Job drawing, mm, ordinate dimensions from the low corner. One solid piece. A direction names the side the tool comes from. Give positions to 0.01 mm unless a question says otherwise; leave off trailing zeros. Loops run counter-clockwise (first coordinate to the right, second up) from the corner with the lowest first, then second, coordinate; pieces in that order, holes last. Notation, with made-up numbers: (-24, 25) -> (-2, 25) arc R26 cw to (-2, 46) -> close; hole circle Ø2 at (41, 42). An arc over 180 degrees is marked (long way). Use one line per item in the form item = value.
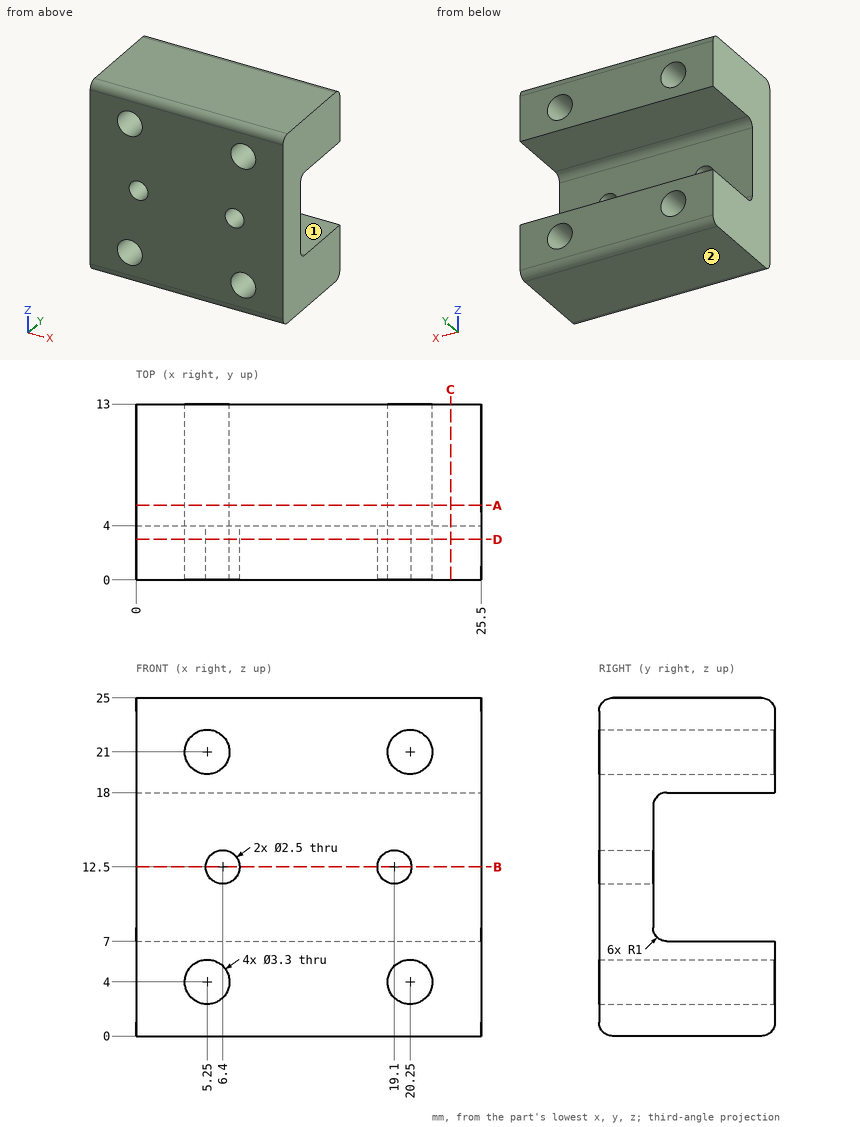
1. Cut at B-B, the plane z = 12.5. Write the cut outline in (x, y), then the cut area to 3 significant figures.
Result sheet:
outline = (0, 0) -> (5.15, 0) -> (5.15, 4) -> (0, 4) -> close; (7.65, 0) -> (17.85, 0) -> (17.85, 4) -> (7.65, 4) -> close; (20.35, 0) -> (25.5, 0) -> (25.5, 4) -> (20.35, 4) -> close
area = 82.0 mm^2
2. Drill centre lines: line 1 (X direction, y = 7, z = 21); line 2 (X direction, y = 12, z = 19.75); line 3 (Z direction, x = 13.5, y = 5.75). Where is each one in solid material? Low to high.
Result sheet:
line_1 = 0 to 3.6, 6.9 to 18.6, 21.9 to 25.5
line_2 = 0 to 4.17, 6.33 to 19.17, 21.33 to 25.5
line_3 = 0 to 7, 18 to 25
3. Cut at A-A, the plane y = 5.5. Write the cut outline in (x, z).
Result sheet:
outline = (0, 0) -> (25.5, 0) -> (25.5, 7) -> (0, 7) -> close; (0, 18) -> (25.5, 18) -> (25.5, 25) -> (0, 25) -> close; hole circle Ø3.3 at (5.25, 4); hole circle Ø3.3 at (5.25, 21); hole circle Ø3.3 at (20.25, 4); hole circle Ø3.3 at (20.25, 21)
4. Tool access for the marked faces 1 and 2: list every direction of +Z, -Z, +X, -X, +Y, -Y with a clear straight run to the whole face (end or side of a thin tool).
Result sheet:
face_1 = +X, -X, +Y
face_2 = -Z, +X, -X, +Y, -Y
5. Cut at C-C, the plane x = 23.25. Write the cut outline in (y, z).
Result sheet:
outline = (0, 1) arc R1 ccw to (1, 0) -> (12, 0) arc R1 ccw to (13, 1) -> (13, 7) -> (5, 7) arc R1 cw to (4, 8) -> (4, 17) arc R1 cw to (5, 18) -> (13, 18) -> (13, 24) arc R1 ccw to (12, 25) -> (1, 25) arc R1 ccw to (0, 24) -> close
6. Drop flat-ended pins along their axis: P1, Ø2.5, axis at x = 5.25, z = 4, coming from the -Y side; P2, Ø1.5, axis at x = 9.5, z = 16.5, coming from the +Y side; P3, Ø7, axis at x = 8, z = 14, coming from the +Y side. Give the stop position or say it passes through.
Result sheet:
P1 = through
P2 = 4.03
P3 = 4.13
7. Cut at D-D, the plane y = 3. Write the cut outline in (x, z).
Result sheet:
outline = (0, 0) -> (25.5, 0) -> (25.5, 25) -> (0, 25) -> close; hole circle Ø3.3 at (5.25, 4); hole circle Ø3.3 at (5.25, 21); hole circle Ø2.5 at (6.4, 12.5); hole circle Ø2.5 at (19.1, 12.5); hole circle Ø3.3 at (20.25, 4); hole circle Ø3.3 at (20.25, 21)
